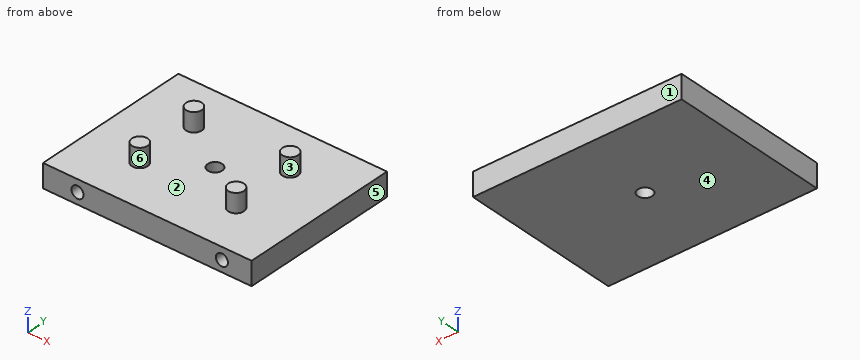
from build123d import *

# Parameters (mm, degrees)
F0_W     = 165.1
F0_H     = 127
F0_R     = 5.715
F1_DEPTH = 18.542
F2_R     = 6.223
F3_DEPTH = 14.859
F4_R     = 4.7625
F5_DEPTH = 65.3288


with BuildPart() as f1:
    # F0 (on Top) → F1 (new body)
    with BuildSketch(Plane.XY):
        with Locations((82.55, 63.5)):
            Rectangle(F0_W, F0_H)
        with Locations((82.55, 63.5)):
            Circle(F0_R, mode=Mode.SUBTRACT)
    extrude(amount=F1_DEPTH)

    # F2 (on face) → F3 (join)
    with BuildSketch(Plane.XY.offset(18.542)):
        with Locations((44.45, 88.9)):
            Circle(F2_R)
        with Locations((120.65, 88.9)):
            Circle(F2_R)
        with Locations((120.65, 38.1)):
            Circle(F2_R)
        with Locations((44.45, 38.1)):
            Circle(F2_R)
    extrude(amount=F3_DEPTH)

    # F4 (on face) → F5 (cut)
    with BuildSketch(Plane.XZ):
        with Locations((27.28341, 9.017)):
            Circle(F4_R)
        with Locations((141.58341, 9.017)):
            Circle(F4_R)
    extrude(amount=-F5_DEPTH, mode=Mode.SUBTRACT)


solid = f1.part
Geometry check sheet. Reference: the model listing, model coordinates, mm. Face numbers are marked on the shaded views. A direction names the side the tool comes from. Give positions to 0.01 mm unless a question says otherwise; leave off trailing zeros. Order: outer loops, then holes, each group sorted by start corner. A loop starts at its lowest first (then second) coordinate and runs counter-clockwise, first axis right, second up. Notation, with made-up numbers: (81, 27) - (120, 27) arc R12 cw to (120, 49) - close; hole circle Ø7 at (3.25, 87). An arc over 180 degrees is marked (long way). Use one line per item in the form item = value.
1) Sectioned sample at D-D (y = 88.9). Record the boundary of the cut face in (x, z).
Working result:
outline = (0, 0) - (165.1, 0) - (165.1, 18.54) - (126.87, 18.54) - (126.87, 33.4) - (114.43, 33.4) - (114.43, 18.54) - (50.67, 18.54) - (50.67, 33.4) - (38.23, 33.4) - (38.23, 18.54) - (0, 18.54) - close
2) Sectioned sample at A-A (y = 63.5). Record the boundary of the cut face in (x, z) (1 decimal).
Working result:
outline = (0, 0) - (76.8, 0) - (76.8, 18.5) - (0, 18.5) - close; (88.3, 0) - (165.1, 0) - (165.1, 18.5) - (88.3, 18.5) - close; hole circle Ø9.5 at (27.3, 9); hole circle Ø9.5 at (141.6, 9)
3) Sectioned sample at B-B (z = 30). Record the boundary of the cut face in (x, y), and give its area (3 significant figures).
Working result:
outline = circle Ø12.45 at (44.45, 38.1); circle Ø12.45 at (44.45, 88.9); circle Ø12.45 at (120.65, 38.1); circle Ø12.45 at (120.65, 88.9)
area = 487 mm^2
4) Material ranges on probe 1 along Z at (x, y) = (14.5, 115); probe 2 along X at (y, z) = (37.5, 23); probe 3 along Y at (x, z) = (41, 23.5), recorded low to high. Write a range as from..to.
Working result:
probe_1 = 0..18.54
probe_2 = 38.26..50.64, 114.46..126.84
probe_3 = 32.92..43.28, 83.72..94.08
5) Depth check by flat-ended pin: pin 1 Ø6 at (x, y) = (117.5, 20.5) entering from +Z; pin 2 Ø5 at (x, z) = (28.5, 7.5) entering from -Y; pin 3 Ø4 at (y, z) = (93.5, 21) entering from -X. Enter the tip coordinate at first touch or a pass-through.
Working result:
pin_1 = 18.54
pin_2 = 65.33
pin_3 = 38.8
6) Draft check along X on the marked faces 3, 4, 5 and 6. Enter one of: released by +X, released by -X, zero draft, split by the parting line, or undercut.
Working result:
face_3 = undercut
face_4 = zero draft
face_5 = released by +X
face_6 = undercut
7) Access from +Z, -Z, +X, -X, +Y, -Y to the whole of each face (thin tool, end or side, straight path). Record for the marked faces 1 and 2.
Working result:
face_1 = +Z, -Z, +X, -X, +Y
face_2 = +Z
8) Sectioned sample at C-C (x = 120.65). Record the boundary of the cut face in (y, z), and give its area (3 significant figures).
Working result:
outline = (0, 0) - (127, 0) - (127, 18.54) - (95.12, 18.54) - (95.12, 33.4) - (82.68, 33.4) - (82.68, 18.54) - (44.32, 18.54) - (44.32, 33.4) - (31.88, 33.4) - (31.88, 18.54) - (0, 18.54) - close
area = 2,720 mm^2
